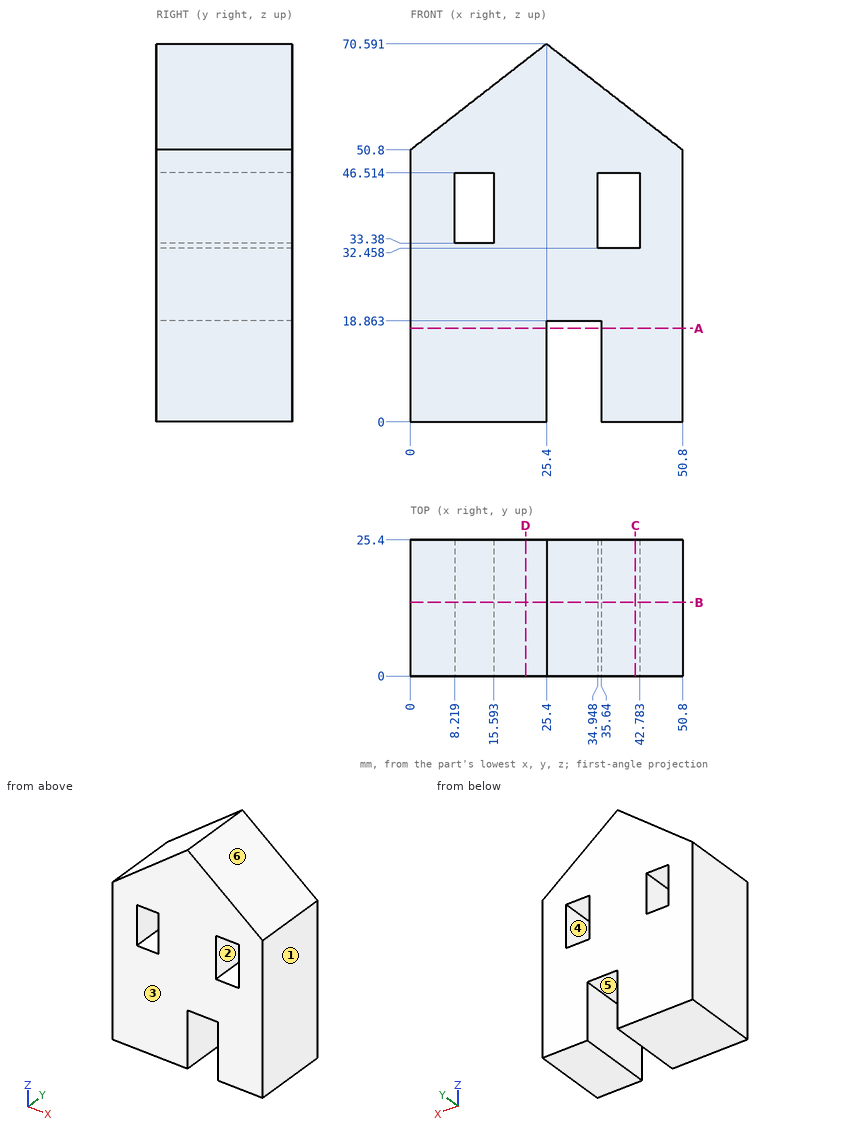
Drawing for the job (mm, zero at the part's lowest x, y, z). A direction names the side the tool comes from. Give positions to 0.01 mm unless a question says otherwise; leave off trailing zeros. Order: outer loops, then holes, each group sorted by start corner. A loop starts at its lowest first (then second) coordinate and runs counter-clockwise, first axis right, second up. Notation, with made-up numbers: M 32.5,28 L 78.5,28 A13 ccw 78.5,47 Z; hole C 40.25,-38.75 d9. An arc over 180 degrees is marked long. Put each result on its own line as item: value. Start each with the question number.
(1) Which spindle directions (+Z, -Z, +X, -X, +Y, -Y) get a long thin tool onto all of the face, cutting with end or side? Do the marked faces 4, 5 and 6. Say none if no direction does.
(2) Flat gauge pins, fed straight in: pin 1 Ø8 at (y, z) = (22, 62.5) entering from +X; pin 2 Ø3 at (x, y) = (30, 12) entering from -Z; pin 3 Ø8.5 at (x, y) = (41, 8) entering from +Z. Where does each tip first touch, or does it go through?
(3) Saw through at A-A, the plane z = 17.5. Write the cut outline in (x, y), then the cut area to 3 significant figures.
(4) Mould opens along X. For the marked faces 1, 2 and 3 say: +X half, -X half, draft (parallel to the pull), parting line (faces both ways), or undercut.
(5) Saw through at D-D, the plane x = 21.5. Write the cut outline in (y, z).
(6) Saw through at C-C, the plane x = 42. Write the cut outline in (y, z).
(7) Saw through at B-B, the plane y = 13.75. Write the cut outline in (x, z).
(8) Drill centre lines: line 1 along X through (y, z) = (2.25, 46); line 2 along X through (y, z) = (24, 16); line 3 along Z through (x, y) = (8.5, 19.75) (1 decimal). Where is each one in solid material? Low to high.
Check result:
1. face 4: +Y, -Y
1. face 5: -Z, +Y, -Y
1. face 6: +Z, +X, +Y, -Y
2. pin 1: stops at x = 40.92
2. pin 2: stops at z = 18.86
2. pin 3: stops at z = 61.75
3. outline: M 0,0 L 25.4,0 L 25.4,25.4 L 0,25.4 Z; M 35.64,0 L 50.8,0 L 50.8,25.4 L 35.64,25.4 Z
3. area: 1,030 mm2
4. face 1: +X half
4. face 2: undercut
4. face 3: draft
5. outline: M 0,0 L 25.4,0 L 25.4,67.55 L 0,67.55 Z
6. outline: M 0,0 L 25.4,0 L 25.4,32.46 L 0,32.46 Z; M 0,46.51 L 25.4,46.51 L 25.4,57.66 L 0,57.66 Z
7. outline: M 0,0 L 25.4,0 L 25.4,18.86 L 35.64,18.86 L 35.64,0 L 50.8,0 L 50.8,50.8 L 25.4,70.59 L 0,50.8 Z; hole M 8.22,33.38 L 15.59,33.38 L 15.59,46.51 L 8.22,46.51 Z; hole M 34.95,32.46 L 42.78,32.46 L 42.78,46.51 L 34.95,46.51 Z
8. line 1: x = 0 to 8.22, 15.59 to 34.95, 42.78 to 50.8
8. line 2: x = 0 to 25.4, 35.64 to 50.8
8. line 3: z = 0 to 33.4, 46.5 to 57.4
